Autodesk Inventor part; units mm, degrees
ref_plane "YZ Plane" through (0, 0, 0) normal (1, 0, 0) x (0, 1, 0)
ref_plane "XZ Plane" through (0, 0, 0) normal (0, 1, 0) x (-1, 0, 0)
ref_plane "XY Plane" through (0, 0, 0) normal (0, 0, 1) x (1, 0, 0)
sketch "Sketch1" plane through (0, 0, 0) normal (0, 1, 0) x (-1, 0, 0)
  line L0 (0.0001, 0.003) -> (0.0001, 0)
  line L1 (0.0001, -17.064) -> (-0.002, -0.0021)
  line L2 (-2.3966, -2.4008) -> (-2.3966, -14.6631)
  line L3 (-2.3966, -14.6631) -> (-6.8866, -14.6631)
  spline S0 degree 3 poles (-6.8866, -14.6631) (-7.1334, -14.6502) (-7.3283, -14.4466) (-7.3261, -14.1977) knots 2 2 2 2 3 3 3 3
  line L4 (-6.8866, -14.6631) -> (-7.1334, -14.6502) construction
  line L5 (-7.1334, -14.6502) -> (-7.3283, -14.4466) construction
  line L6 (-7.3283, -14.4466) -> (-7.3261, -14.1977) construction
  line L7 (-7.2677, -7.2678) -> (-4.8517, -7.2677)
  line L8 (-9.7961, -9.7964) -> (-12.2057, -9.7985)
  line L9 (-4.8515, -9.7963) -> (-9.7961, -9.7964)
  line L10 (-4.8515, -12.2081) -> (-4.8515, -9.7963)
  line L11 (-7.3261, -12.2103) -> (-4.8515, -12.2081)
  line L12 (-7.3261, -14.1977) -> (-7.3261, -12.2103)
  line L13 (-12.2057, -9.7985) -> (-12.206, -12.2102)
  line L14 (-17.0619, -17.062) -> (0.0001, -17.064)
  line L15 (-12.206, -12.2102) -> (-9.7379, -12.2102)
  line L16 (-9.7379, -12.2102) -> (-9.7379, -14.228)
  line L17 (-9.7379, -14.228) -> (-9.7509, -14.4705) construction
  spline S1 degree 3 poles (-9.7379, -14.228) (-9.7509, -14.4705) (-9.9544, -14.661) (-10.2034, -14.6631) knots 11 11 11 11 12 12 12 12
  line L18 (-9.7509, -14.4705) -> (-9.9544, -14.661) construction
  line L19 (-9.9544, -14.661) -> (-10.2034, -14.6631) construction
  line L20 (-14.6632, -14.6631) -> (-14.6675, -14.6631)
  line L21 (-10.2034, -14.6631) -> (-14.6632, -14.6631)
  line L22 (-17.064, 0.0001) -> (-17.0619, -17.062)
  line L23 (-12.206, -7.2698) -> (-7.2677, -7.2678)
  line L24 (-14.6675, -14.6631) -> (-14.6676, -2.4008)
  line L25 (-12.206, -4.8538) -> (-12.206, -7.2698)
  line L26 (-9.7357, -2.8642) -> (-9.738, -4.8538)
  line L27 (-9.738, -4.8538) -> (-12.206, -4.8538)
  line L28 (-9.7357, -2.6174) -> (-9.7357, -2.8642) construction
  spline S2 degree 3 poles (-10.1731, -2.4009) (-9.9285, -2.4159) (-9.7357, -2.6174) (-9.7357, -2.8642) knots 16 16 16 16 17 17 17 17
  line L29 (-10.1731, -2.4009) -> (-9.9285, -2.4159) construction
  line L30 (-9.9285, -2.4159) -> (-9.7357, -2.6174) construction
  line L31 (-14.6676, -2.4008) -> (-10.1731, -2.4009)
  line L32 (-0.002, -0.0021) -> (0.0001, 0)
  line L33 (0.0001, 0) -> (-17.064, 0.0001)
  line L34 (-4.8517, -7.2677) -> (-4.8516, -4.8558)
  line L35 (-7.3282, -4.8559) -> (-7.3282, -2.8294)
  line L36 (-4.8536, -4.8537) -> (-7.3282, -4.8559)
  line L37 (-7.3087, -2.5977) -> (-7.1248, -2.4138) construction
  spline S3 degree 3 poles (-7.3282, -2.8294) (-7.3087, -2.5977) (-7.1248, -2.4138) (-6.893, -2.3986) knots 26 26 26 26 27 27 27 27
  line L38 (-7.3282, -2.8294) -> (-7.3087, -2.5977) construction
  line L39 (-7.1248, -2.4138) -> (-6.893, -2.3986) construction
  line L40 (-4.8516, -4.8558) -> (-4.8536, -4.8537)
  line L41 (-6.893, -2.3986) -> (-2.3985, -2.3986)
  line L42 (-2.3985, -2.3986) -> (-2.3964, -2.4007)
  line L43 (-2.3964, -2.4007) -> (-2.3966, -2.4008)
  line L44 (15.402, -0.0001) -> (-1.6922, 0)
  dimension "d2" = 17.0942
extrude "Extrusion1" add sketch "Sketch1" along normal blind 0.254
properties part number "Logo Inlay"
Input: part model. Units: mm. Frame: model coordinates. Give positions to 0.01 mm unless a question says otherwise; leave off trailing zeros. Write each loop counter-clockwise with the first axis right and the second up, starting at its lowest first coordinate (ties: lowest second). Pieces come first, ordered by that corner, then holes. Notation, with made-up numbers: M 55,-28 L 87,-28 A35 ccw 87,7 Z; hole C 57,11 d3. An arc over 180 degrees is marked long. Use one line per item in the form item = value.
1. Cut plane A-A on x = 6.5. Return loops of the section in (y, z), and give its area (3 significant figures).
Outcome:
outline = M 0,-17.06 L 0.25,-17.06 L 0.25,-14.66 L 0,-14.66 Z; M 0,-12.21 L 0.25,-12.21 L 0.25,-9.8 L 0,-9.8 Z; M 0,-7.27 L 0.25,-7.27 L 0.25,-4.86 L 0,-4.86 Z; M 0,-2.4 L 0.25,-2.4 L 0.25,0 L 0,0 Z
area = 2.44 mm²
2. First-contact query: P1, Ø2, axis at x = 11, z = -14.5, coming from the -Y side. Flat tip, straight axial feed; report the tip coordinate or a pass-through.
Outcome:
P1 = 0
3. Cut plane D-D on z = -7.5. Return loops of the section in (x, y), and give its area (3 significant figures).
Outcome:
outline = M 0,0 L 2.4,0 L 2.4,0.25 L 0,0.25 Z; M 14.67,0 L 17.06,0 L 17.06,0.25 L 14.67,0.25 Z
area = 1.22 mm²
4. Cut plane C-C on z = -4. Return loops of the section in (x, y), and give its area (3 significant figures).
Outcome:
outline = M 0,0 L 2.4,0 L 2.4,0.25 L 0,0.25 Z; M 7.33,0 L 9.74,0 L 9.74,0.25 L 7.33,0.25 Z; M 14.67,0 L 17.06,0 L 17.06,0.25 L 14.67,0.25 Z
area = 1.83 mm²
5. Cut plane B-B on x = 8.75. Return loops of the section in (y, z), and give its area (3 significant figures).
Outcome:
outline = M 0,-17.06 L 0.25,-17.06 L 0.25,-9.8 L 0,-9.8 Z; M 0,-7.27 L 0.25,-7.27 L 0.25,0 L 0,0 Z
area = 3.69 mm²
6. Ray query, L1, parallel to X at y = 0.1, z = -13; L2, parallel to X at y = 0.1, z = -6.25; L3, parallel to Z at x = 10.5, y = 0.1. Return the intervals inside material, ascending.
Outcome:
L1 = 0 to 2.4, 7.33 to 9.74, 14.67 to 17.06
L2 = 0 to 2.4, 4.85 to 12.21, 14.67 to 17.06
L3 = -17.06 to -14.66, -12.21 to -9.8, -7.27 to -4.85, -2.4 to 0
